The figure shows three views and two pictorial views of one solid part (mm, origin at its lowest corner). Answer the questions. Coordinates: 2 decimals unless noted, no trailing zeros. Order: outer loops, then holes, each group sorted by start corner. A loop starts at its lowest first (then second) coordinate and runs counter-clockwise, first axis right, second up. Notation, with made-up numbers: (77.5, 86.25) -> (126.5, 86.25) arc R23 ccw to (126.5, 94.25) -> close; hole circle Ø11 at (-28, 70). An arc over 180 degrees is marked (long way). Use one line per item in the form item = value.
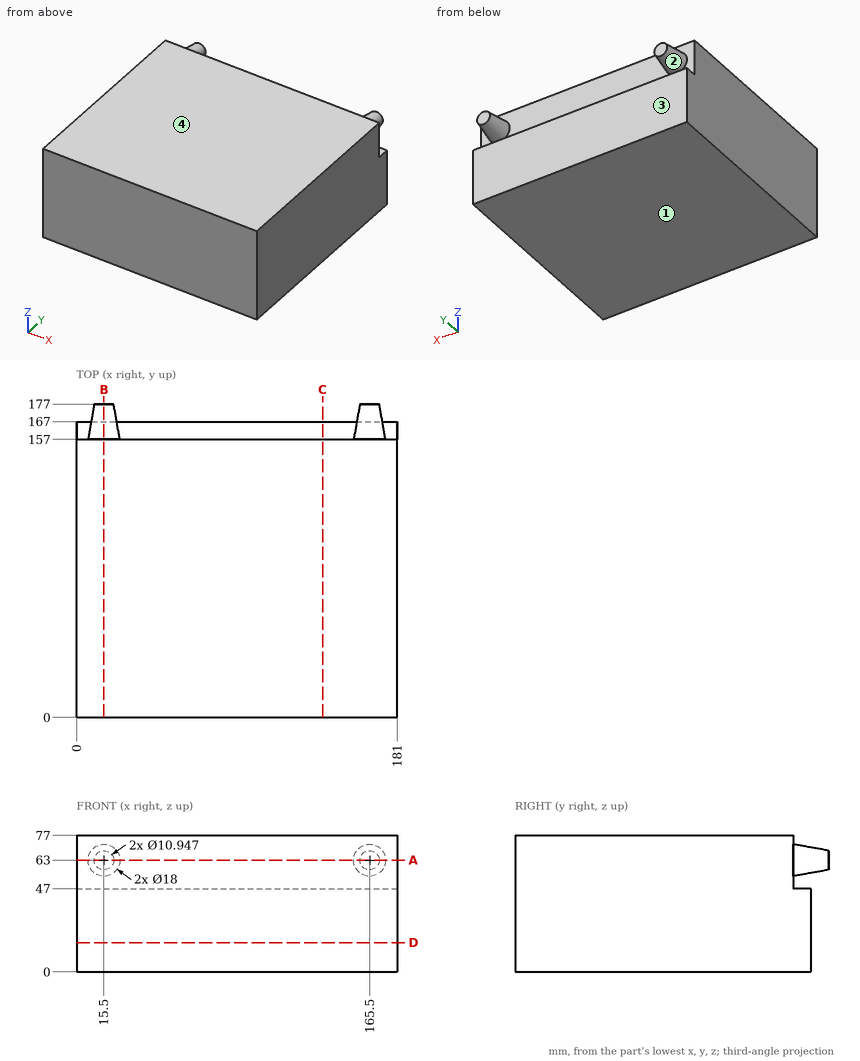
(1) Section B-B on x = 15.5 is taken. Write down the section's boundary in (y, z), plus the area to 3 significant figures.
Data:
outline = (0, 0) -> (167, 0) -> (167, 47) -> (157, 47) -> (157, 54) -> (177, 57.53) -> (177, 68.47) -> (157, 72) -> (157, 77) -> (0, 77) -> close
area = 12,800 mm²
(2) Straight lines are drawn through the part: line 1 along Y through (x, z) = (84, 60); line 2 along Y through (x, z) = (108.5, 4); line 3 along Z through (x, y) = (63, 164). For each, find the intervals that lie inside material, in ascending order.
Data:
line_1 = 0 to 157
line_2 = 0 to 167
line_3 = 0 to 47
(3) Section C-C on x = 139 is taken. Write down the section's boundary in (y, z).
Data:
outline = (0, 0) -> (167, 0) -> (167, 47) -> (157, 47) -> (157, 77) -> (0, 77) -> close
(4) Each of these flat-tipped pins is pushed along its axis until it touches: P1, Ø10, axis at x = 66, z = 33, coming from the +Y side; P2, Ø5, axis at x = 86, y = 164, coming from the +Z side; P3, Ø9, axis at x = 52.5, z = 68, coming from the +Y side. Where does it stop, or does it pass through?
Data:
P1 = 167
P2 = 47
P3 = 157
(5) Section A-A on z = 63 is taken. Write down the section's boundary in (x, y).
Data:
outline = (0, 0) -> (181, 0) -> (181, 157) -> (174.5, 157) -> (170.97, 177) -> (160.03, 177) -> (156.5, 157) -> (24.5, 157) -> (20.97, 177) -> (10.03, 177) -> (6.5, 157) -> (0, 157) -> close
(6) The mould has two halves that part along Z. Classify the marked faces 1, 2, 3 and 4: released by +Z, released by -Z, zero draft, split by the parting line, or undercut.
Data:
face_1 = released by -Z
face_2 = undercut
face_3 = zero draft
face_4 = released by +Z
(7) Section D-D on z = 16.5 is taken. Write down the section's boundary in (x, y), plus the area to 3 significant figures.
Data:
outline = (0, 0) -> (181, 0) -> (181, 167) -> (0, 167) -> close
area = 30,200 mm²
